The listing builds one solid part. Answer for the finished solid, in the listing's coordinates (mm). Round coordinates to 2 decimals unless told otherwise and drop trailing zeros. Order: outer loops, then holes, each group sorted by start corner. A loop starts at its lowest first (then second) coordinate and runs counter-clockwise, first axis right, second up. Notation, with made-up numbers: (64, 28.5) -> (78, 28.5) arc R35 ccw to (78, 64.5) -> close; hole circle Ø4 at (50.25, 86). An arc over 180 degrees is marked (long way). Return JSON: item names as keys, results as strings. Group by question number.
(1) Consider line 1 (X direction, y = 105.5, z = 6.25); line 2 (Y direction, x = -19, z = 1); line 3 (Y direction, x = 20, z = 8). Determine where each line is inside the solid, lowest interval first. Write a range as [from, to].
(2) The part is cut by section A-A (z = 2.5). Count the separate pieces of the cut face and the enclosed holes in it, plus the area to 3 significant figures.
(3) Determine the mould class of faces 1 (the face through (14.14, 111.46, 2.96)), 2 (the face through (-23.65, 131.126, 4.93)), 3 (the face through (-3, 71, 10)) for opening direction Y: +Y half, -Y half, draft (parallel to the pull), parting line (faces both ways), or undercut.
(4) Each of these flat-tipped pins is pushed along its axis until it touches: pin 1 (14.5 mm diameter, centred on x = -20.28, y = 107, fed in from +Z); pin 2 (11.5 mm diameter, centred on x = -20.28, y = 33, fed in from +Z). Where does it stop, or does it pass through?
(5) The part is cut by section C-C (y = 16.5). Determine the outline of the cut face in (x, z), plus the area to 3 significant figures.
(6) The part is cut by section B-B (y = 107). Determine the outline of the cut face in (x, z), plus the area to 3 significant figures.
from build123d import *

# Parameters (mm, degrees)
F0_W     = 60
F0_H     = 140
F0_R     = 4.5
F0_R_2   = 2.75
F1_DEPTH = 10
F2_SIZE  = 4
F3_SIZE  = 18


with BuildPart() as f1:
    # F0 (on Top) → F1 (new body)
    with BuildSketch(Plane.XY):
        with Locations((-2.776433, 70)):
            Rectangle(F0_W, F0_H)
        with Locations((-20.276433, 33)):
            Circle(F0_R, mode=Mode.SUBTRACT)
        with Locations((-17.076433, 18)):
            Circle(F0_R_2, mode=Mode.SUBTRACT)
        with Locations((11.523567, 18)):
            Circle(F0_R_2, mode=Mode.SUBTRACT)
        with Locations((14.723567, 33)):
            Circle(F0_R, mode=Mode.SUBTRACT)
        with Locations((-20.276433, 107)):
            Circle(F0_R, mode=Mode.SUBTRACT)
        with Locations((-17.076433, 122)):
            Circle(F0_R_2, mode=Mode.SUBTRACT)
        with Locations((11.523567, 122)):
            Circle(F0_R_2, mode=Mode.SUBTRACT)
        with Locations((14.723567, 107)):
            Circle(F0_R, mode=Mode.SUBTRACT)
    extrude(amount=F1_DEPTH)

    # F2
    f2_edges = [f1.edges().sort_by_distance(p)[0] for p in [
        (-24.776433, 33, 10),
        (10.223567, 33, 10),
        (10.223567, 107, 10),
        (-24.776433, 107, 10),
    ]]
    chamfer(f2_edges, length=F2_SIZE)

    # F3
    f3_edges = [f1.edges().sort_by_distance(p)[0] for p in [
        (-32.776433, 0, 5),
        (27.223567, 0, 5),
        (27.223567, 140, 5),
        (-32.776433, 140, 5),
    ]]
    chamfer(f3_edges, length=F3_SIZE)


solid = f1.part
Answer below:
{
 "1": {"line 1": "x = [-32.78, -24.78], [-15.77, 10.22], [19.23, 27.22]", "line 2": "y = [4.22, 16.03], [19.97, 28.68], [37.32, 102.68], [111.32, 120.03], [123.97, 135.78]", "line 3": "y = [10.78, 29.2], [36.8, 103.2], [110.8, 129.22]"},
 "2": {"separate pieces": "1", "enclosed holes": "8", "area": "7,400 mm²"},
 "3": {"face 1": "undercut", "face 2": "+Y half", "face 3": "draft"},
 "4": {"pin 1": "stops at z = 8.75", "pin 2": "stops at z = 7.25"},
 "5": {"outline": "(-31.28, 0) -> (-19.38, 0) -> (-19.38, 10) -> (-31.28, 10) -> close; (-14.77, 0) -> (9.22, 0) -> (9.22, 10) -> (-14.77, 10) -> close; (13.83, 0) -> (25.72, 0) -> (25.72, 10) -> (13.83, 10) -> close", "area": "478 mm²"},
 "6": {"outline": "(-32.78, 0) -> (-24.78, 0) -> (-24.78, 6) -> (-28.78, 10) -> (-32.78, 10) -> close; (-15.78, 0) -> (10.22, 0) -> (10.22, 6) -> (6.22, 10) -> (-11.78, 10) -> (-15.78, 6) -> close; (19.22, 0) -> (27.22, 0) -> (27.22, 10) -> (23.22, 10) -> (19.22, 6) -> close", "area": "388 mm²"}
}
